Verification items for the finished model (mm, model axes). Face numbers are marked on the shaded views. A direction names the side the tool comes from. Coordinates: 2 decimals unless noted, no trailing zeros. Write each loop counter-clockwise with the first axis right and the second up, starting at its lowest first coordinate (ties: lowest second). Pieces come first, ordered by that corner, then holes. Notation, with made-up numbers: (69.25, -37.75) -> (91.25, -37.75) arc R17 ccw to (91.25, -7.75) -> close; hole circle Ø7 at (0.25, 5). An arc over 180 degrees is marked (long way). Use a Markdown table: item, result. Add a question column.
from build123d import *

# Parameters (mm, degrees)
SKETCH2_W               = 5
SKETCH2_H               = 1
SKETCH2_W_2             = 1
SKETCH2_H_2             = 5
CUT_EXTRUDE_THIN1_DEPTH = 0.5
FILLET2_R               = 0.125


with BuildPart() as part:
    # Sketch1 → Revolve1 (revolve)
    with BuildSketch(Plane.XY, mode=Mode.PRIVATE) as revolve1_sk:
        Polygon((0, 0), (0, -0.79375), (1.5875, -0.79375), (1.5875, -7.14375), (3.175, -7.14375), (3.175, 0), align=None)
    revolve(revolve1_sk.sketch.rotate(Axis((3.175, -7.14375, 0), (0, 1, 0)), 270), axis=Axis((3.175, -7.14375, 0), (0, 1, 0)))

    # Sketch2 → Cut-Extrude-Thin1 (cut)
    with BuildSketch(Plane(origin=(0, 0, 0), x_dir=(1, 0, 0), z_dir=(0, 1, 0))):
        with Locations((3.175, 0)):
            Rectangle(SKETCH2_W, SKETCH2_H)
        with Locations((3.175, 0)):
            Rectangle(SKETCH2_W_2, SKETCH2_H_2)
    extrude(amount=-CUT_EXTRUDE_THIN1_DEPTH, mode=Mode.SUBTRACT)

    # Fillet2
    fillet2_edges = [part.edges().sort_by_distance(p)[0] for p in [
        (4.675, -0.5, 0.5),
        (1.675, -0.5, 0.5),
        (1.675, -0.5, -0.5),
        (3.175, -0.5, -2.5),
        (3.675, -0.5, -1.5),
        (4.675, -0.5, -0.5),
        (5.675, -0.5, 0),
        (3.675, -0.5, 1.5),
        (3.175, -0.5, 2.5),
        (0.675, -0.5, 0),
        (2.675, -0.5, -1.5),
        (2.675, -0.5, 1.5),
    ]]
    fillet(fillet2_edges, radius=FILLET2_R)


solid = part.part
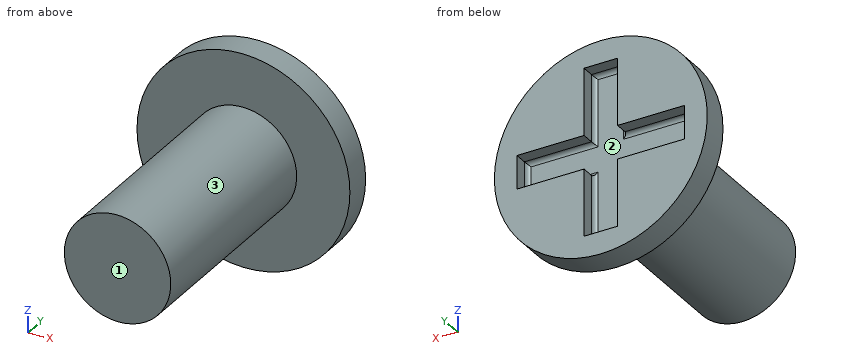
1) Cross-section at D-D on z = -1. Record the boundary of the cut face in (x, y) (3 decimals), then the cut area to 3 significant figures.
2) Thickness scan on L1, parallel to Y at x = 5.5, z = -1.5; L2, parallel to Y at x = 5, z = 0; L3, parallel to Z at x = 3.25, y = -6.5. Record the ranges inside material, lowest first.
3) Cross-section at C-C on y = -4.5. Record the boundary of the cut face in (x, z) (1 decimal).
4) Cross-section at B-B on x = 5. Record the boundary of the cut face in (y, z) (3 decimals).
5) Gauge pin test, flat ends, axial feed: pin 1 (1 mm diameter, centred on x = 1.5, z = -1.5, fed in from -Y); pin 2 (1 mm diameter, centred on x = 1.5, y = -5.5, fed in from +Z); pin 3 (1 mm diameter, centred on y = -4, z = 0, fed in from -X). Record the tip position at first contact, or that the pin passes through.
6) Set-up check for the marked faces 1, 2 and 3: record each of +Z, -Z, +X, -X, +Y, -Y from which the full face is reachable in a straight line by a thin tool's end or side.
Returned:
| question | item | result |
|---|---|---|
| 1 | outline | (0.162, -0.794) -> (1.942, -0.794) -> (1.942, -7.144) -> (4.408, -7.144) -> (4.408, -0.794) -> (6.188, -0.794) -> (6.188, 0) -> (3.675, 0) -> (3.675, -0.375) arc R0.125 cw to (3.55, -0.5) -> (2.8, -0.5) arc R0.125 cw to (2.675, -0.375) -> (2.675, 0) -> (0.162, 0) -> close |
| 1 | area | 19.9 mm² |
| 2 | L1 | y = -0.79 to 0 |
| 2 | L2 | y = -0.79 to -0.5 |
| 2 | L3 | z = -1.59 to 1.59 |
| 3 | outline | circle Ø3.2 at (3.2, 0) |
| 4 | outline | (-0.794, -2.598) -> (0, -2.598) -> (0, -0.5) -> (-0.375, -0.5) arc R0.125 cw to (-0.5, -0.375) -> (-0.5, 0.375) arc R0.125 cw to (-0.375, 0.5) -> (0, 0.5) -> (0, 2.598) -> (-0.794, 2.598) -> close |
| 5 | pin 1 | stops at y = -0.79 |
| 5 | pin 2 | stops at z = 1.07 |
| 5 | pin 3 | stops at x = 1.59 |
| 6 | face 1 | +Z, -Z, +X, -X, -Y |
| 6 | face 2 | +Y |
| 6 | face 3 | -Y |
